from build123d import *

# Parameters (mm, degrees)
SKETCH1_W           = 27
SKETCH1_H           = 10
BOSS_EXTRUDE1_DEPTH = 3
SKETCH5_R           = 3
BOSS_EXTRUDE3_DEPTH = 3
SKETCH6_R           = 1.5
CUT_EXTRUDE1_DEPTH  = 3
SKETCH7_R           = 4
CUT_EXTRUDE2_DEPTH  = 2
SKETCH8_R           = 3.5
CUT_EXTRUDE4_DEPTH  = 41.635575547


with BuildPart() as part:
    # Sketch1 → Boss-Extrude1 (new body)
    with BuildSketch(Plane(origin=(0, 0, 0), x_dir=(1, 0, 0), z_dir=(0, 1, 0))):
        Rectangle(SKETCH1_W, SKETCH1_H)
    boss_extrude1 = extrude(amount=BOSS_EXTRUDE1_DEPTH)

    # Sketch5 → Boss-Extrude3 (add)
    with BuildSketch(Plane(origin=(13.5, 0, 0), x_dir=(0, 0, -1), z_dir=(1, 0, 0))):
        with BuildLine():
            Line((-5, 3), (5, 3))
            Line((5, 3), (5, 36))
            ThreePointArc((5, 36), (0, 41), (-5, 36))
            Line((-5, 36), (-5, 3))
        make_face()
        with Locations((0, 36)):
            Circle(SKETCH5_R, mode=Mode.SUBTRACT)
    boss_extrude3 = extrude(amount=-BOSS_EXTRUDE3_DEPTH)

    # Sketch6 → Cut-Extrude1 (cut)
    with BuildSketch(Plane(origin=(0, 3, 0), x_dir=(1, 0, 0), z_dir=(0, 1, 0))):
        with Locations(Location((0, 0, 0), (0, 0, 270))):
            Circle(SKETCH6_R)
    extrude(amount=-CUT_EXTRUDE1_DEPTH, mode=Mode.SUBTRACT)

    # Sketch7 → Cut-Extrude2 (cut)
    with BuildSketch(Plane.ZY.offset(-10.5)):
        with Locations((0, 36)):
            Circle(SKETCH7_R)
    cut_extrude2 = extrude(amount=-CUT_EXTRUDE2_DEPTH, mode=Mode.SUBTRACT)

    # Mirror3: Boss-Extrude1, Boss-Extrude3, Cut-Extrude2 across plane
    add(boss_extrude1.mirror(Plane(origin=(0, 0, 0), x_dir=(0, 0, 1), z_dir=(1, 0, 0))))
    add(boss_extrude3.mirror(Plane(origin=(0, 0, 0), x_dir=(0, 0, 1), z_dir=(1, 0, 0))))
    add(cut_extrude2.mirror(Plane(origin=(0, 0, 0), x_dir=(0, 0, 1), z_dir=(1, 0, 0))), mode=Mode.SUBTRACT)

    # Sketch8 → Cut-Extrude4 (cut, through all)
    with BuildSketch(Plane(origin=(0, 3, 0), x_dir=(1, 0, 0), z_dir=(0, 1, 0))):
        with Locations(Location((0, 0, 0), (0, 0, 270))):
            Circle(SKETCH8_R)
    extrude(amount=-CUT_EXTRUDE4_DEPTH, mode=Mode.SUBTRACT)


solid = part.part
Work out the finished part from the listing and answer in its coordinate system (mm). A direction names the side the tool comes from. Round coordinates to 2 decimals unless told otherwise and drop trailing zeros. Write each loop counter-clockwise with the first axis right and the second up, starting at its lowest first coordinate (ties: lowest second). Pieces come first, ordered by that corner, then holes. Notation, with made-up numbers: M 9.25,75 L 41.25,75 A31 cw 41.25,111 Z; hole C 59,87.5 d6. An arc over 180 degrees is marked long. Use a Markdown table: item, result.
1) The part is cut by section B-B on z = 0. Give the vertices of the cut face in (x, y), plus the area to 3 significant figures.
Taken from the geometry:
| item | result |
|---|---|
| outline | M -13.5,0 L -3.5,0 L -3.5,3 L -10.5,3 L -10.5,32 L -12.5,32 L -12.5,33 L -13.5,33 Z; M -13.5,39 L -12.5,39 L -12.5,40 L -10.5,40 L -10.5,41 L -13.5,41 Z; M 3.5,0 L 13.5,0 L 13.5,33 L 12.5,33 L 12.5,32 L 10.5,32 L 10.5,3 L 3.5,3 Z; M 10.5,40 L 12.5,40 L 12.5,39 L 13.5,39 L 13.5,41 L 10.5,41 Z |
| area | 244 mm2 |
2) Determine the mould class of faces 4 (the face through (10.5, 18, 0)), 5 (the face through (11.486, 39.966, -0.521)), 6 (the face through (12.5, 39, 1)), 7 (the face through (12, 41, 0)) for opening direction Z: pulls with the +Z half, pulls with the -Z half, needs draft (parallel to the pull), parting line crosses it, or undercut.
Taken from the geometry:
| item | result |
|---|---|
| face 4 | needs draft |
| face 5 | undercut |
| face 6 | undercut |
| face 7 | parting line crosses it |
3) A flat-ended cylindrical pin translates along its axis: pin 1 (5 mm diameter, centred on x = 2.5, z = 0.5, fed in from +Y). Find the tip coordinate at first contact, or state that the pin passes through.
Taken from the geometry:
| item | result |
|---|---|
| pin 1 | stops at y = 3 |
4) Consider line 1 (X direction, y = 26.5, z = -1); line 2 (Y direction, x = -11.45, z = 0); line 3 (Y direction, x = 4.25, z = -1.5). Determine where each line is inside the solid, lowest interval first. Write a range as [from, to].
Taken from the geometry:
| item | result |
|---|---|
| line 1 | x = [-13.5, -10.5], [10.5, 13.5] |
| line 2 | y = [0, 32], [40, 41] |
| line 3 | y = [0, 3] |
5) Which of the six approach directions +Z, -Z, +X, -X, +Y, -Y give full straight-line access (tool end or side, diameter ignored) to faces 1 (the face through (-10.5, 18, 0)), 2 (the face through (-12.5, 39, 1)), 3 (the face through (-13, 39, 0))?
Taken from the geometry:
| item | result |
|---|---|
| face 1 | +Z, -Z, +Y |
| face 2 | none |
| face 3 | +X, -X |
6) The part is cut by section D-D on x = 11.75. Give the vertices of the cut face in (y, z), plus the area to 3 significant figures.
Taken from the geometry:
| item | result |
|---|---|
| outline | M 0,-5 L 36,-5 A5 ccw 36,5 L 0,5 Z; hole C 36,0 d8 |
| area | 349 mm2 |
7) The part is cut by section C-C on x = 0. Give the vertices of the cut face in (y, z).
Taken from the geometry:
| item | result |
|---|---|
| outline | M 0,-5 L 3,-5 L 3,-3.5 L 0,-3.5 Z; M 0,3.5 L 3,3.5 L 3,5 L 0,5 Z |
8) The part is cut by section A-A on y = 25. Give the vertices of the cut face in (x, z).
Taken from the geometry:
| item | result |
|---|---|
| outline | M -13.5,-5 L -10.5,-5 L -10.5,5 L -13.5,5 Z; M 10.5,-5 L 13.5,-5 L 13.5,5 L 10.5,5 Z |
